Geometry check sheet. Reference: the model listing, model coordinates, mm. Face numbers are marked on the shaded views. A direction names the side the tool comes from. Give positions to 0.01 mm unless a question says otherwise; leave off trailing zeros. Loops run counter-clockwise (first coordinate to the right, second up) from the corner with the lowest first, then second, coordinate; pieces in that order, holes last.
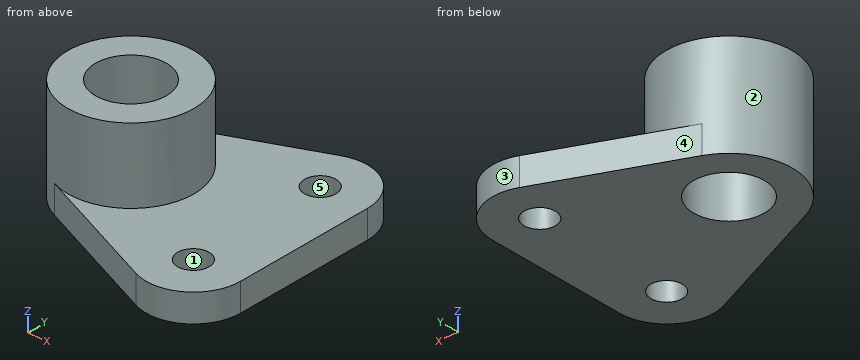
```python
from build123d import *
from build123d import SkipClean  # not in build123d's __all__

# Parameters (mm, degrees)
F0_R     = 14.2875
F0_R_2   = 6.35
F1_DEPTH = 11.176
F2_DEPTH = 41.148
F3_DEPTH = 11.177
F4_DEPTH = 41.149


with BuildPart() as f1:
    # F0 (on Top) → F1 (new body)
    with BuildSketch(Plane.XY):
        with BuildLine():
            ThreePointArc((-61.399120046, 23.3629201096), (-37.4323475039, 21.1933093342), (-26.0324774843, 0))
            ThreePointArc((-26.0324774843, 0), (-37.4323475039, -21.1933093342), (-61.399120046, -23.3629201096))
            Line((-61.399120046, -23.3629201096), (-8.1074594056, -46.0971900822))
            ThreePointArc((-8.1074594056, -46.0971900822), (-11.1325749696, -12.6800179994), (18.4175225157, -28.575))
            Line((18.4175225157, -28.575), (18.4175225157, 28.575))
            ThreePointArc((18.4175225157, 28.575), (-11.1325749696, 12.6800179994), (-8.1074594056, 46.0971900822))
            Line((-8.1074594056, 46.0971900822), (-61.399120046, 23.3629201096))
        make_face()
        with BuildLine():
            ThreePointArc((-61.399120046, -23.3629201096), (-37.4323475039, -21.1933093342), (-26.0324774843, 0))
            ThreePointArc((-26.0324774843, 0), (-37.4323475039, 21.1933093342), (-61.399120046, 23.3629201096))
            ThreePointArc((-61.399120046, 23.3629201096), (-76.8324774843, 0), (-61.399120046, -23.3629201096))
        make_face()
        with Locations((-51.4324774843, 0)):
            Circle(F0_R, mode=Mode.SUBTRACT)
        with BuildLine():
            ThreePointArc((18.4175225157, 28.575), (9.867620001, 44.4699820006), (-8.1074594056, 46.0971900822))
            ThreePointArc((-8.1074594056, 46.0971900822), (-11.1325749696, 12.6800179994), (18.4175225157, 28.575))
        make_face()
        with Locations((-0.6324774843, 28.575)):
            Circle(F0_R_2, mode=Mode.SUBTRACT)
        with BuildLine():
            ThreePointArc((18.4175225157, -28.575), (-11.1325749696, -12.6800179994), (-8.1074594056, -46.0971900822))
            ThreePointArc((-8.1074594056, -46.0971900822), (9.867620001, -44.4699820006), (18.4175225157, -28.575))
        make_face()
        with Locations((-0.6324774843, -28.575)):
            Circle(F0_R_2, mode=Mode.SUBTRACT)
        with Locations((-51.4324774843, 0)):
            Circle(F0_R)
        with Locations((-0.6324774843, -28.575)):
            Circle(F0_R_2)
        with Locations((-0.6324774843, 28.575)):
            Circle(F0_R_2)
    extrude(amount=F1_DEPTH)

    # F0 (on Top) → F2 (join)
    with BuildSketch(Plane.XY):
        with BuildLine():
            ThreePointArc((-61.399120046, -23.3629201096), (-37.4323475039, -21.1933093342), (-26.0324774843, 0))
            ThreePointArc((-26.0324774843, 0), (-37.4323475039, 21.1933093342), (-61.399120046, 23.3629201096))
            ThreePointArc((-61.399120046, 23.3629201096), (-76.8324774843, 0), (-61.399120046, -23.3629201096))
        make_face()
        with Locations((-51.4324774843, 0)):
            Circle(F0_R, mode=Mode.SUBTRACT)
    with SkipClean():  # cleaning this boolean's faces spoils the solid; the shape is the same uncleaned
        extrude(amount=F2_DEPTH)

    # F3 (cut, through all): a face of the model
    f3_faces = [f1.faces().sort_by_distance(p)[0] for p in [
        (-51.4324774843, 0, 11.176),
    ]]
    with SkipClean():  # cleaning this boolean's faces spoils the solid; the shape is the same uncleaned
        extrude(f3_faces, amount=-F3_DEPTH, mode=Mode.SUBTRACT)

    # F0 (on Top) → F4 (cut, through all)
    with BuildSketch(Plane.XY):
        with Locations((-0.6324774843, 28.575)):
            Circle(F0_R_2)
        with Locations((-0.6324774843, -28.575)):
            Circle(F0_R_2)
    with SkipClean():  # cleaning this boolean's faces spoils the solid; the shape is the same uncleaned
        extrude(amount=F4_DEPTH, mode=Mode.SUBTRACT)


solid = f1.part
```
1) Sectioned sample at B-B on z = 4. Count the separate pieces of the cut face and the enclosed holes in it, plus the area to 3 significant figures.
2) Sectioned sample at D-D on x = -29. Enter the section's corners in (y, z), plus the area to 3 significant figures.
3) Sectioned sample at A-A on y = 0. Enter the section's corners in (x, z), plus the area to 3 significant figures.
4) Mould release check, pull along X, two halves, no side actions. Record for the marked faces 3, 4 and 5: +X half, -X half, draft (parallel to the pull), parting line (faces both ways), or undercut.
5) Depth check by flat-ended pin: P1, Ø2, axis at x = -43, z = 26.5, coming from the -Y side. Enter the tip coordinate at first touch or a pass-through.
6) Scan lines: line 1 along X through (y, z) = (-1, 7); line 2 along X through (y, z) = (27.5, 10); line 3 along Z through (x, y) = (4.5, -5). Record each from-to range of solid material in increasing order.
7) Tool access check on the marked faces 1 and 2. Record the directions out of +Z, -Z, +X, -X, +Y, -Y that give a thin tool (end or side, any length) a straight path to the whole face; none if there is none.
8) Sectioned sample at C-C on x = -54.5. Enter the section's corners in (y, z).
Determined:
1. separate pieces: 1
1. enclosed holes: 3
1. area: 5,690 mm2
2. outline: (-37.18, 0) - (37.18, 0) - (37.18, 11.18) - (11.91, 11.18) - (11.91, 41.15) - (-11.91, 41.15) - (-11.91, 11.18) - (-37.18, 11.18) - close
2. area: 1,550 mm2
3. outline: (-76.83, 0) - (-65.72, 0) - (-65.72, 41.15) - (-76.83, 41.15) - close; (-37.14, 0) - (18.42, 0) - (18.42, 11.18) - (-26.03, 11.18) - (-26.03, 41.15) - (-37.14, 41.15) - close
3. area: 1,410 mm2
4. face 3: parting line
4. face 4: -X half
4. face 5: undercut
5. P1: stops at y = -24.29
6. line 1: x = -76.81 to -65.68, -37.18 to 18.42
6. line 2: x = -51.7 to -6.89, 5.63 to 18.42
6. line 3: z = 0 to 11.18
7. face 1: +Z, -Z
7. face 2: +Z
8. outline: (-26.31, 0) - (-13.95, 0) - (-13.95, 41.15) - (-25.21, 41.15) - (-25.21, 11.18) - (-26.31, 11.18) - close; (13.95, 0) - (26.31, 0) - (26.31, 11.18) - (25.21, 11.18) - (25.21, 41.15) - (13.95, 41.15) - close
